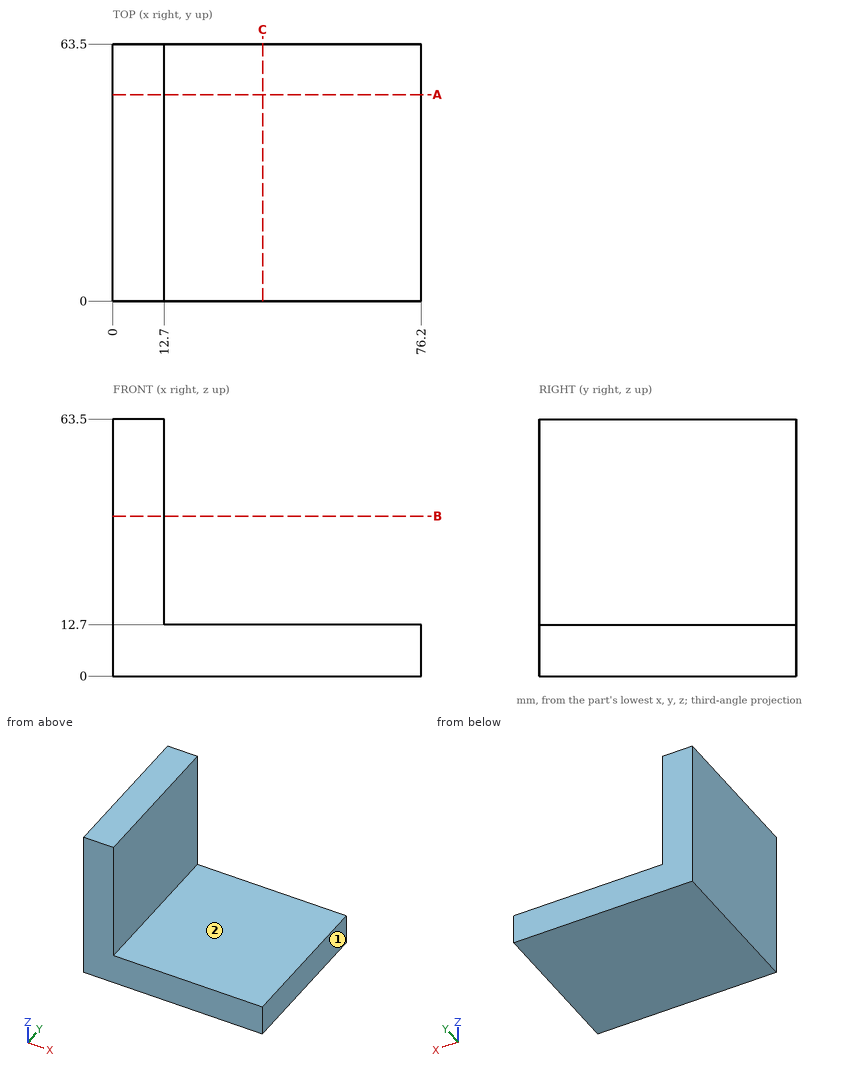
Verification items for this drawing (mm, ordinates from the low corner). A direction names the side the tool comes from. Round coordinates to 2 decimals unless told otherwise and drop trailing zeros. Order: outer loops, then holes, each group sorted by start corner. A loop starts at its lowest first (then second) coordinate and runs counter-clockwise, first axis right, second up. Notation, with made-up numbers: (15.25, -19) - (23.25, -19) arc R20 cw to (23.25, 16) - close; hole circle Ø4 at (68.25, 47.25). An arc over 180 degrees is marked (long way). Use CSV: the item, a comma, the result in double quotes. Start each with the question number.
1) Section check C-C, the plane x = 37. Record the cut outline in (y, z), plus the area to 3 significant figures.
2) Access from +Z, -Z, +X, -X, +Y, -Y to the whole of each face (thin tool, end or side, straight path). Record for the marked faces 1 and 2.
3) Section check B-B, the plane z = 39.5. Record the cut outline in (x, y), plus the area to 3 significant figures.
4) Section check A-A, the plane y = 51. Record the cut outline in (x, z), plus the area to 3 significant figures.
5) Go/stop test with flat-tipped pins: P1, Ø5, axis at x = 63.5, y = 13, coming from the +Z side; P2, Ø12, axis at x = 21.5, z = 29, coming from the +Y side; P3, Ø1.5, axis at x = 54.5, y = 22.5, coming from the -Z side. Record where each tip stops, or that it passes through.
6) Thickness scan on L1, parallel to Z at x = 32.5, y = 52. Record the ranges inside material, lowest first.
Answers:
1,outline,"(0, 0) - (63.5, 0) - (63.5, 12.7) - (0, 12.7) - close"
1,area,"806 mm²"
2,face 1,"+Z, -Z, +X, +Y, -Y"
2,face 2,"+Z, +X, +Y, -Y"
3,outline,"(0, 0) - (12.7, 0) - (12.7, 63.5) - (0, 63.5) - close"
3,area,"806 mm²"
4,outline,"(0, 0) - (76.2, 0) - (76.2, 12.7) - (12.7, 12.7) - (12.7, 63.5) - (0, 63.5) - close"
4,area,"1,610 mm²"
5,P1,"stops at z = 12.7"
5,P2,"passes through"
5,P3,"stops at z = 0"
6,L1,"z = 0 to 12.7"
